Input: part model. Units: mm. Frame: model coordinates. Coordinates: 2 decimals unless noted, no trailing zeros. Write each loop counter-clockwise with the first axis right and the second up, starting at its lowest first coordinate (ties: lowest second). Pieces come first, ordered by that corner, then holes. Notation, with made-up numbers: (-27, 76.5) - (4, 76.5) arc R14 ccw to (4, 82.5) - close; hole circle Ø3 at (0.5, 17.5). An arc over 180 degrees is marked (long way). Put each result on its own line as item: value. Start each with the question number.
1. Pin query (flat end, axial travel): pin 1 (3 mm diameter, centred on x = 11, y = 2, fed in from -Z); pin 2 (0.6 mm diameter, centred on x = 1, y = 0.5, fed in from -Z); pin 3 (1.5 mm diameter, centred on y = 0, z = 0, fed in from -X). Return the tip coordinate at first contact, or that it passes through.
2. Cut plane A-A, the plane x = 1.5. Return loops of the section in (y, z), and give its area (3 significant figures).
3. Line query: line 1 (X direction, y = -2.5, z = 1.5); line 2 (X direction, y = -0.25, z = -1); line 3 (Y direction, x = 10, z = 1.25). Output: solid intervals per line, ascending.
from build123d import *

# Parameters (mm, degrees)
FILLET1_R       = 0.3048
HEX_2_DEPTH     = 1.9558
THDSCHPAT_COUNT = 24
THDSCHPAT_PITCH = 0.76073


with BuildPart() as part:
    # BodySke → Base-Revolve (revolve)
    with BuildSketch(Plane.XY):
        Polygon((0, 0), (0, 3.0226), (0.4064, 3.429), (4.1656, 3.429), (4.1656, 2.0828), (22.74316, 2.0828), (23.2156, 1.61036), (23.2156, 0), align=None)
    revolve(axis=Axis((-31.75, 0, 0), (1, 0, 0)))

    # Fillet1
    fillet1_edges = [part.edges().sort_by_distance(p)[0] for p in [
        (4.1656, -2.0828, 0),
    ]]
    fillet(fillet1_edges, radius=FILLET1_R)

    # Sketch2 → Hex-PreBroach (revolve, cut)
    with BuildSketch(Plane.XY):
        Polygon((0, 1.778), (1.9558, 1.778), (2.982328779, 0), (0, 0), align=None)
    revolve(axis=Axis((0, 0, 0), (1, 0, 0)), mode=Mode.SUBTRACT)

    # Sketch3 → Hex 2 (cut)
    with BuildSketch(Plane(origin=(0, 0, 0), x_dir=(0, 0.5, 0.866025404), z_dir=(-1, 0, 0))):
        Polygon((1.026528779, 1.778), (-1.026528779, 1.778), (-2.053057557, 0), (-1.026528779, -1.778), (1.026528779, -1.778), (2.053057557, 0), align=None)
    extrude(amount=-HEX_2_DEPTH, mode=Mode.SUBTRACT)

    # ThdSchSke → ThreadSchematic (revolve, cut)
    with BuildSketch(Plane.XY):
        Polygon((4.95808, -1.61036), (4.627273951, -2.0828), (4.627273951, -2.6035), (5.288886049, -2.6035), (5.288886049, -2.0828), align=None)
    threadschematic = revolve(axis=Axis((-3.175, 0, 0), (1, 0, 0)), mode=Mode.SUBTRACT)

    # ThdSchPat: ThreadSchematic ×24
    with Locations(*[(i * THDSCHPAT_PITCH, 0, 0) for i in range(1, THDSCHPAT_COUNT)]):
        add(threadschematic, mode=Mode.SUBTRACT)


solid = part.part
Report:
1. pin 1: stops at z = -2.01
1. pin 2: stops at z = -3.42
1. pin 3: stops at x = 2.55
2. outline: circle Ø6.86 at (0, 0); hole (-2.05, 0) - (-1.03, -1.78) - (1.03, -1.78) - (2.05, 0) - (1.03, 1.78) - (-1.03, 1.78) - close
2. area: 26.0 mm^2
3. line 1: x = 0 to 4.17
3. line 2: x = 2.39 to 23.22
3. line 3: y = -1.58 to 1.58
